Input: part model. Units: mm. Frame: model coordinates. Face numbers are marked on the shaded views. A direction names the side the tool comes from. Round coordinates to 2 decimals unless told otherwise and drop trailing zeros. Loops run counter-clockwise (first coordinate to the right, second up) from the corner with the lowest first, then second, coordinate; pieces in that order, holes last. Notation, with made-up numbers: (19, 36.25) -> (27, 36.25) arc R19 ccw to (27, 60.25) -> close; hole circle Ø9 at (0, 32). An arc over 180 degrees is marked (long way). Answer as a JSON object with one key per item and string values.
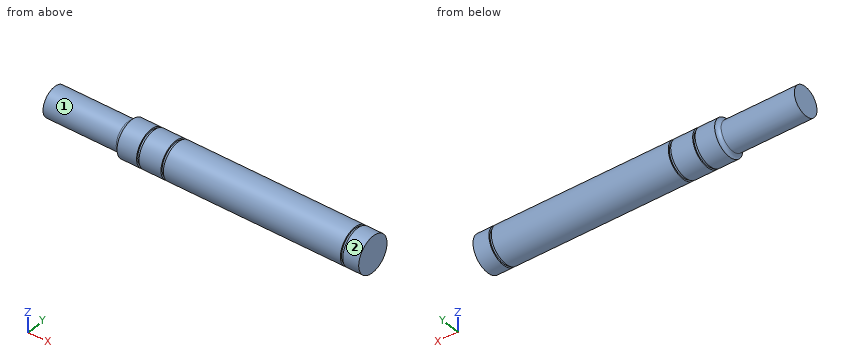
```python
from build123d import *


with BuildPart() as part:
    # Sketch1 → Revolve1 (revolve)
    with BuildSketch(Plane(origin=(0, 0, 0), x_dir=(-1, 0, 0), z_dir=(0, 0, 1)), mode=Mode.PRIVATE) as revolve1_sk:
        with BuildLine():
            Line((93.245668053, 287.354869365), (93.245668053, 287.754869365))
            Line((93.245668053, 287.754869365), (87.245668053, 287.754869365))
            Line((87.245668053, 287.754869365), (87.245668053, 287.354869365))
            Line((87.245668053, 287.354869365), (86.585668053, 287.354869365))
            Line((86.585668053, 287.354869365), (86.585668053, 287.754869365))
            Line((86.585668053, 287.754869365), (38.245668053, 287.754869365))
            Line((38.245668053, 287.754869365), (38.245668053, 287.354869365))
            Line((38.245668053, 287.354869365), (37.585668053, 287.354869365))
            Line((37.585668053, 287.354869365), (37.585668053, 287.754869365))
            Line((37.585668053, 287.754869365), (33.245668053, 287.754869365))
            Line((33.245668053, 287.754869365), (33.245668053, 282.754869365))
            Line((33.245668053, 282.754869365), (120.245668053, 282.754869365))
            Line((120.245668053, 282.754869365), (120.245668053, 286.754869365))
            Line((120.245668053, 286.754869365), (100.245668053, 286.754869365))
            ThreePointArc((100.245668053, 286.754869365), (99.538561272, 287.047762584), (99.245668053, 287.754869365))
            Line((99.245668053, 287.754869365), (93.905668053, 287.754869365))
            Line((93.905668053, 287.754869365), (93.905668053, 287.354869365))
            Line((93.905668053, 287.354869365), (93.245668053, 287.354869365))
        make_face()
    revolve(revolve1_sk.sketch.rotate(Axis((-33.245668053, -282.754869365, 0), (-1, 0, 0)), 270), axis=Axis((-33.245668053, -282.754869365, 0), (-1, 0, 0)))


solid = part.part
```
1) Section C-C, the plane x = -90. Output: boundary loops of the cut face in (y, z), plus the area to 3 significant figures.
Output:
{"outline": "circle Ø10 at (-282.75, 0)", "area": "78.5 mm^2"}
2) Contact query for flat-ended pins moving along their axis: P1, Ø6, axis at x = -111, z = -1.5, coming from the -Y side; P2, Ø6, axis at x = -109, z = -1, coming from the +Y side; P3, Ø5, axis at x = -55, y = -286.5, coming from the +Z side. Output: stop coordinate, or through.
Output:
{"P1": "stops at y = -286.75", "P2": "stops at y = -278.75", "P3": "stops at z = 4.84"}
3) Ray query, probe 1 along X at (y, z) = (-280.75, 4.25); probe 2 along Z at (x, y) = (-56, -282.5); probe 3 along Y at (x, z) = (-99, 3). Return the intervals inside material, ascending.
Output:
{"probe 1": "x = -99.29 to -93.91, -93.25 to -87.25, -86.59 to -38.25, -37.59 to -33.25", "probe 2": "z = -4.99 to 4.99", "probe 3": "y = -286.75 to -278.75"}
4) Section B-B, the plane x = -106.5. Output: boundary loops of the cut face in (y, z), plus the area to 3 significant figures.
Output:
{"outline": "circle Ø8 at (-282.75, 0)", "area": "50.3 mm^2"}
5) Reachability of the marked faces 1 and 2 from +Z, -Z, +X, -X, +Y, -Y: full face, straight path, thin tool, end or side. Return the list, or none.
Output:
{"face 1": "-X", "face 2": "+X, -X"}
